Design review of the part built by this model. Coordinates are the model's own, in mm. Give positions to 0.01 mm unless a question says otherwise; leave off trailing zeros. Order: outer loops, then holes, each group sorted by start corner. A loop starts at its lowest first (then second) coordinate and runs counter-clockwise, first axis right, second up. Notation, with made-up numbers: M 45,71.5 L 59,71.5 A32 cw 59,100.5 Z; hole C -33,-20 d1. An arc over 180 degrees is marked long. Answer as a JSON object with one key per item and string values.
Autodesk Inventor part; units mm, degrees
ref_plane "YZ Plane" through (0, 0, 0) normal (1, 0, 0) x (0, 1, 0)
ref_plane "XZ Plane" through (0, 0, 0) normal (0, 1, 0) x (-1, 0, 0)
ref_plane "XY Plane" through (0, 0, 0) normal (0, 0, 1) x (1, 0, 0)
sketch "Sketch1" plane through (0, 0, 0) normal (0, 1, 0) x (-1, 0, 0)
  circle A0 centre (0, 0) radius 5
  dimension "d0" = 10
extrude "Extrusion1" add sketch "Sketch1" along normal blind 12
sketch "Sketch2" plane through (0, 0, 0) normal (1, 0, 0) x (0, 1, 0)
  line L0 (1.5, -2.5) -> (2.5, -2.5)
  line L1 (2.5, -2.5) -> (2.5, -7.5)
  line L2 (2.5, -7.5) -> (1.5, -7.5)
  line L3 (1.5, -7.5) -> (1.5, -2.5)
  line L4 (0, -5) -> (12, -5)
  line L5 (1.5, -2.5) -> (2.5, -7.5) construction
  line L6 (2.5, -2.5) -> (1.5, -7.5) construction
  line L7 (0, 0) -> (12, 0)
  line L8 (12, -5) -> (12, 5)
  line L9 (0, -10) -> (0, 7.5)
  line L10 (-2.4, 0) -> (14.4, 0)
  point P0 (2, -5)
  dimension "d3" = 1
  dimension "d4" = 5
  dimension "d9" = 2
revolve "Revolution1" cut sketch "Sketch2" angle 360 about axis through (0, 0, 0) along (0, 1, 0) contours L0 L1 L4 L3 | L4 L1 L2 L3
pattern_linear "Rectangular Pattern1" count 5 spacing 2 along (0, 1, 0) of "Revolution1"
properties part number "Ceramic_Spacer"
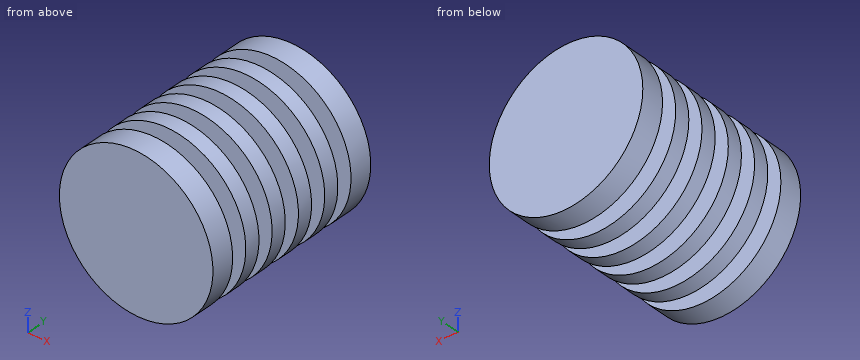
(1) We need section A-A (z = -3). Write out the cut boundary in (x, y).
Checked values:
{"outline": "M -4,0 L 4,0 L 4,1.5 L -4,1.5 Z; M -4,2.5 L 4,2.5 L 4,3.5 L -4,3.5 Z; M -4,4.5 L 4,4.5 L 4,5.5 L -4,5.5 Z; M -4,6.5 L 4,6.5 L 4,7.5 L -4,7.5 Z; M -4,8.5 L 4,8.5 L 4,9.5 L -4,9.5 Z; M -4,10.5 L 4,10.5 L 4,12 L -4,12 Z"}
(2) To check wall thickness, follow L1, parallel to Y at x = -1, z = 4; L2, parallel to X at y = 2.25, z = 0.5; L3, parallel to Z at x = -0.75, y = 6. State the ranges of each line that lie inside material, in increasing order. Write a range as from..to.
Checked values:
{"L1": "y = 0..1.5, 2.5..3.5, 4.5..5.5, 6.5..7.5, 8.5..9.5, 10.5..12", "L2": "x = -2.45..2.45", "L3": "z = -2.38..2.38"}
(3) We need section B-B (x = 3.5). Write out the cut boundary in (y, z), plus the area to 3 significant figures.
Checked values:
{"outline": "M 0,-3.57 L 1.5,-3.57 L 1.5,3.57 L 0,3.57 Z; M 2.5,-3.57 L 3.5,-3.57 L 3.5,3.57 L 2.5,3.57 Z; M 4.5,-3.57 L 5.5,-3.57 L 5.5,3.57 L 4.5,3.57 Z; M 6.5,-3.57 L 7.5,-3.57 L 7.5,3.57 L 6.5,3.57 Z; M 8.5,-3.57 L 9.5,-3.57 L 9.5,3.57 L 8.5,3.57 Z; M 10.5,-3.57 L 12,-3.57 L 12,3.57 L 10.5,3.57 Z", "area": "50.0 mm^2"}
(4) We need section D-D (y = 10.75). Write out the cut boundary in (x, z).
Checked values:
{"outline": "C 0,0 d10"}
(5) We need section C-C (y = 3.75). Write out the cut boundary in (x, z), plus the area to 3 significant figures.
Checked values:
{"outline": "C 0,0 d5", "area": "19.6 mm^2"}
(6) Insertion check: pin 1 (1.5 mm diameter, centred on y = 7.5, z = 2.5, fed in from -X); pin 2 (1.5 mm diameter, centred on y = 4, z = -3, fed in from -X); pin 3 (2 mm diameter, centred on x = -3, y = 7, fed in from +Z). Each pin has a flat end and moves straight along its axis. Give the tip position at first contact, or say it passes through.
Checked values:
{"pin 1": "stops at x = -4.68", "pin 2": "stops at x = -4.36", "pin 3": "stops at z = 4.58"}
